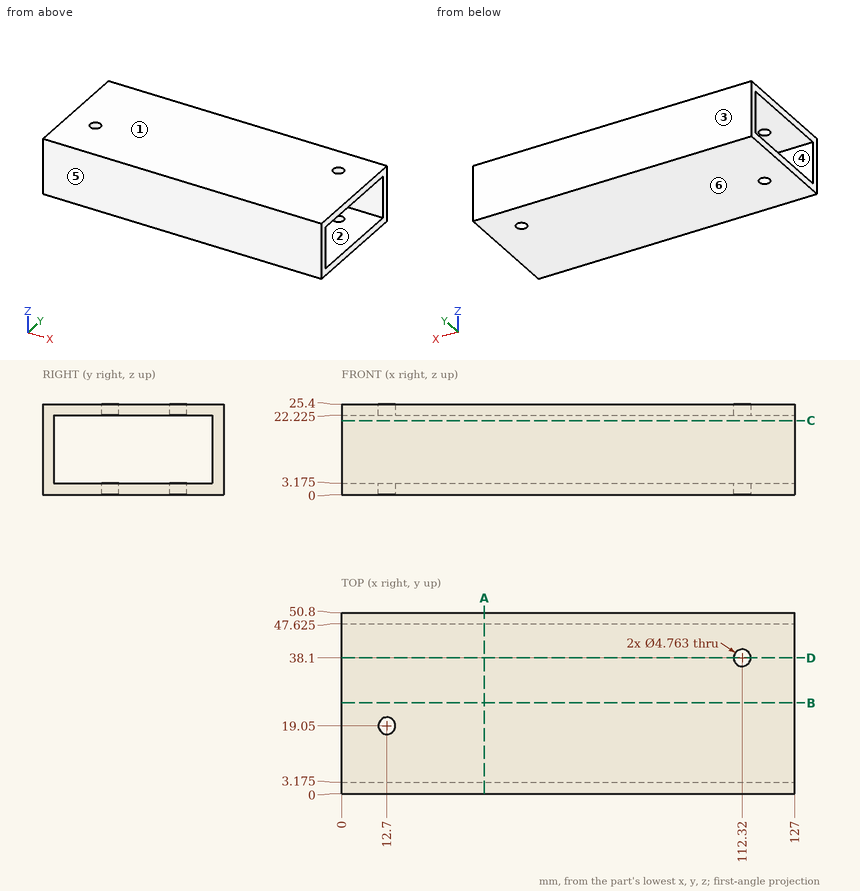
Study the drawing (mm; zero at the part's minimum x, y, z) and answer. A direction names the side the tool comes from. Give positions to 0.01 mm unless a question says otherwise; leave off trailing zeros. Write each loop counter-clockwise with the first axis right and the second up, starting at its lowest first coordinate (ties: lowest second). Pieces come first, ordered by that corner, then holes. Notation, with made-up numbers: (-15.75, -31) - (31.25, -31) arc R15 ccw to (31.25, -14) - close; hole circle Ø5 at (40.25, -20.5). An arc over 180 degrees is marked (long way). Use CSV: the item, a comma, the result in double quotes. Start each with the question number.
(1) Find section C-C (z = 20.75). Give the vertices of the cut face in (x, y) (1 decimal).
(2) Find section B-B (y = 25.5). Give the vertices of the cut face in (x, z) (1 decimal).
(3) For the marked faces 1 and 2, determine the directions among +Z, -Z, +X, -X, +Y, -Y from which every point of the face is accessible in a straight line to the end or side of a thin tool.
(4) Find section D-D (y = 38.1). Give the vertices of the cut face in (x, z) (1 decimal).
(5) Determine the mould class of the marked faces 3, 4, 5 and 6 for opening direction Y: +Y half, -Y half, draft (parallel to the pull), parting line (faces both ways), or undercut.
(6) Find section A-A (x = 40). Give the vertices of the cut face in (y, z) (1 decimal).
(7) Consider line 1 along Y through (x, z) = (98, 6.5) (1 decimal); line 2 along Y through (x, z) = (12.7, 23.5); line 3 along Z through (x, y) = (111, 4) (1 decimal). Determine where each line is inside the solid, lowest interval first.
Findings below:
1,outline,"(0, 0) - (127, 0) - (127, 3.2) - (0, 3.2) - close; (0, 47.6) - (127, 47.6) - (127, 50.8) - (0, 50.8) - close"
2,outline,"(0, 0) - (127, 0) - (127, 3.2) - (0, 3.2) - close; (0, 22.2) - (127, 22.2) - (127, 25.4) - (0, 25.4) - close"
3,face 1,"+Z, +X, -X, +Y, -Y"
3,face 2,"+X, -X"
4,outline,"(0, 0) - (109.9, 0) - (109.9, 3.2) - (0, 3.2) - close; (0, 22.2) - (109.9, 22.2) - (109.9, 25.4) - (0, 25.4) - close; (114.7, 0) - (127, 0) - (127, 3.2) - (114.7, 3.2) - close; (114.7, 22.2) - (127, 22.2) - (127, 25.4) - (114.7, 25.4) - close"
5,face 3,"+Y half"
5,face 4,"undercut"
5,face 5,"-Y half"
5,face 6,"draft"
6,outline,"(0, 0) - (50.8, 0) - (50.8, 25.4) - (0, 25.4) - close; hole (3.2, 3.2) - (47.6, 3.2) - (47.6, 22.2) - (3.2, 22.2) - close"
7,line 1,"0 to 3.2, 47.6 to 50.8"
7,line 2,"0 to 16.67, 21.43 to 50.8"
7,line 3,"0 to 3.2, 22.2 to 25.4"
